Can you work these out from the model? Positions are in its coordinate system, mm. A direction names the side the tool comes from. Give positions to 0.01 mm unless a question says otherwise; leave off trailing zeros. Write each loop counter-clockwise with the first axis right and the second up, starting at its lowest first coordinate (ties: lowest second). Pieces come first, ordered by that corner, then holes. Notation, with made-up numbers: (24.25, 31) -> (40.25, 31) arc R29 cw to (40.25, 56) -> close; hole circle Ø8 at (68.25, 17). An arc over 180 degrees is marked (long way). Answer as CSV lines item,"result". Start each with the question number.
1. I'm going to push flat-ended pins straight in: P1, Ø5, axis at x = -3, y = 2.5, coming from the +Z side; P2, Ø1.5, axis at x = 5, z = -4.5, coming from the -Y side; P3, Ø8, axis at y = 10, z = 0, coming from the -X side. Where does each tip first touch, or does it pass through?
2. If we section it at C-C on z = 8: Write out the boundary of the cut face in (x, y), plus the area to 3 significant figures.
3. If we section it at B-B on z = 0: Write out the boundary of the cut face in (x, y).
4. If we mould it in two halves opening along X, with no side actions, what happens to faces 1 (the face through (9.735, 3.274, -0.228)), 2 (the face through (-2, 0, -4)), 3 (the face through (-10.74, 3.23, -2.38))? For each: pulls with the +X half, pulls with the -X half, needs draft (parallel to the pull), parting line crosses it, or undercut.
5. If we section it at A-A on x = 0: Write out the boundary of the cut face in (y, z).
6. If we section it at D-D on y = 10.75: Write out the boundary of the cut face in (x, z).
7. I need wall thicknesses on line 1 (X direction, y = 2.65, z = 0); line 2 (X direction, y = 2.6, z = -8); line 3 (Z direction, x = 1.5, y = 5.25). Which ranges of each line are inside material? Lowest first, please. Write a range as [from, to].
8. On a 3-axis mill with a long thin cutter (end or side, diameter ignored), from which of +Z, -Z, +X, -X, +Y, -Y can I reach the whole of each face in a straight line? I mean faces 4 (the face through (3, 1.5, -5)), 5 (the face through (3, 5, -5)), 6 (the face through (-9.55, 3.27, 0.81)). Say none if no direction works.
```python
from build123d import *

# Parameters (mm, degrees)
SKETCH_1_R          = 5.5
SKETCH_1_R_2        = 4
EXTRUDE_1_DEPTH     = 1.5
SKETCH_2_R          = 11
SKETCH_2_R_2        = 4
EXTRUDE_2_DEPTH     = 3.5
SKETCH_3_R          = 5.5
SKETCH_3_R_2        = 4
EXTRUDE_3_DEPTH     = 10
SKETCH_4_R          = 1.75
CUT_EXTRUDE_1_DEPTH = 19.493242009


with BuildPart() as part:
    # 草图1 → 凸台-拉伸1 (new body)
    with BuildSketch(Plane(origin=(0, 0, 0), x_dir=(1, 0, 0), z_dir=(0, 1, 0))):
        with Locations(Location((0, 0, 0), (0, 0, 270))):
            Circle(SKETCH_1_R)
        with Locations(Location((0, 0, 0), (0, 0, 270))):
            Circle(SKETCH_1_R_2, mode=Mode.SUBTRACT)
    extrude(amount=EXTRUDE_1_DEPTH)

    # 草图2 → 凸台-拉伸2 (add)
    with BuildSketch(Plane(origin=(0, 1.5, 0), x_dir=(1, 0, 0), z_dir=(0, 1, 0))):
        with Locations(Location((0, 0, 0), (0, 0, 270))):
            Circle(SKETCH_2_R)
        with Locations(Location((0, 0, 0), (0, 0, 270))):
            Circle(SKETCH_2_R_2, mode=Mode.SUBTRACT)
    extrude(amount=EXTRUDE_2_DEPTH)

    # 草图3 → 凸台-拉伸3 (add)
    with BuildSketch(Plane(origin=(0, 5, 0), x_dir=(1, 0, 0), z_dir=(0, 1, 0))):
        with Locations(Location((0, 0, 0), (0, 0, 270))):
            Circle(SKETCH_3_R)
        with Locations(Location((0, 0, 0), (0, 0, 270))):
            Circle(SKETCH_3_R_2, mode=Mode.SUBTRACT)
    extrude(amount=EXTRUDE_3_DEPTH)

    # 草图4 → 切除-拉伸1 (cut, through all)
    with BuildSketch(Plane(origin=(0, 5, 0), x_dir=(1, 0, 0), z_dir=(0, 1, 0))):
        with Locations(Location((0, 8, 0), (0, 0, 270))):
            Circle(SKETCH_4_R)
        with Locations(Location((8, 0, 0), (0, 0, 270))):
            Circle(SKETCH_4_R)
        with Locations(Location((0, -8, 0), (0, 0, 270))):
            Circle(SKETCH_4_R)
        with Locations(Location((-8, 0, 0), (0, 0, 270))):
            Circle(SKETCH_4_R)
    extrude(amount=-CUT_EXTRUDE_1_DEPTH, mode=Mode.SUBTRACT)


solid = part.part
```
Computed values:
1,P1,"stops at z = 10.99"
1,P2,"stops at y = 1.5"
1,P3,"stops at x = -5.5"
2,outline,"(-7.55, 1.5) -> (-1.75, 1.5) -> (-1.75, 5) -> (-7.55, 5) -> close; (1.75, 1.5) -> (7.55, 1.5) -> (7.55, 5) -> (1.75, 5) -> close"
2,area,"40.6 mm2"
3,outline,"(-11, 1.5) -> (-9.75, 1.5) -> (-9.75, 5) -> (-11, 5) -> close; (-6.25, 1.5) -> (-5.5, 1.5) -> (-5.5, 0) -> (-4, 0) -> (-4, 15) -> (-5.5, 15) -> (-5.5, 5) -> (-6.25, 5) -> close; (4, 0) -> (5.5, 0) -> (5.5, 1.5) -> (6.25, 1.5) -> (6.25, 5) -> (5.5, 5) -> (5.5, 15) -> (4, 15) -> close; (9.75, 1.5) -> (11, 1.5) -> (11, 5) -> (9.75, 5) -> close"
4,face 1,"undercut"
4,face 2,"needs draft"
4,face 3,"parting line crosses it"
5,outline,"(0, -5.5) -> (1.5, -5.5) -> (1.5, -6.25) -> (5, -6.25) -> (5, -5.5) -> (15, -5.5) -> (15, -4) -> (0, -4) -> close; (0, 4) -> (15, 4) -> (15, 5.5) -> (5, 5.5) -> (5, 6.25) -> (1.5, 6.25) -> (1.5, 5.5) -> (0, 5.5) -> close; (1.5, -11) -> (5, -11) -> (5, -9.75) -> (1.5, -9.75) -> close; (1.5, 9.75) -> (5, 9.75) -> (5, 11) -> (1.5, 11) -> close"
6,outline,"circle Ø11 at (0, 0); hole circle Ø8 at (0, 0)"
7,line 1,"x = [-11, -9.75], [-6.25, -4], [4, 6.25], [9.75, 11]"
7,line 2,"x = [-7.55, -1.75], [1.75, 7.55]"
7,line 3,"z = [-5.29, -3.71], [3.71, 5.29]"
8,face 4,"-Y"
8,face 5,"+Y"
8,face 6,"+Y, -Y"
